```python
from build123d import *

# Parameters (mm, degrees)
F0_R     = 300
F1_DEPTH = 17.1
F3_DEPTH = 2
F4_R     = 4
F5_DEPTH = 25
F6_R     = 48
F7_DEPTH = 6
F8_R     = 15
F9_DEPTH = 11.101


# Not quite as in the source:
# - a feature names something its author has since deleted; it is built from what else it names


with BuildPart() as f1:
    # F0 (on Top) → F1 (new body)
    with BuildSketch(Plane.XY):
        Circle(F0_R)
    extrude(amount=F1_DEPTH)

    # F2 (on face) → F3 (cut)
    with BuildSketch(Plane.XY.offset(17.1)):
        Polygon((-144.8616802798, -16.1682461039), (-263.6556195192, -134.9621853432), (-134.9621853432, -263.6556195192), (-16.1682461039, -144.8616802798), align=None)
        Polygon((144.8616802798, -16.1682461039), (16.1682461039, -144.8616802798), (134.9621853432, -263.6556195192), (263.6556195192, -134.9621853432), align=None)
        Polygon((16.1682461039, 144.8616802798), (144.8616802798, 16.1682461039), (263.6556195192, 134.9621853432), (134.9621853432, 263.6556195192), align=None)
        Polygon((-144.8616802798, 16.1682461039), (-16.1682461039, 144.8616802798), (-134.9621853432, 263.6556195192), (-263.6556195192, 134.9621853432), align=None)
    extrude(amount=-F3_DEPTH, mode=Mode.SUBTRACT)

    # F4 (on face) → F5 (cut)
    with BuildSketch(Plane.XY.offset(17.1)):
        with Locations((-263.6556195192, -99.6068462839)):
            Circle(F4_R)
        with Locations((-99.6068462839, -263.6556195192)):
            Circle(F4_R)
        with Locations((99.6068462839, -263.6556195192)):
            Circle(F4_R)
        with Locations((263.6556195192, -99.6068462839)):
            Circle(F4_R)
        with Locations((263.6556195192, 99.6068462839)):
            Circle(F4_R)
        with Locations((99.6068462839, 263.6556195192)):
            Circle(F4_R)
        with Locations((-99.6068462839, 263.6556195192)):
            Circle(F4_R)
        with Locations((-263.6556195192, 99.6068462839)):
            Circle(F4_R)
    extrude(amount=-F5_DEPTH, mode=Mode.SUBTRACT)

    # F6 (on face) → F7 (cut)
    with BuildSketch(Plane.XY.offset(17.1)):
        Circle(F6_R)
    extrude(amount=-F7_DEPTH, mode=Mode.SUBTRACT)

    # F8 (on face) → F9 (cut, through all)
    with BuildSketch(Plane.XY.offset(11.1)):
        Circle(F8_R)
    extrude(amount=-F9_DEPTH, mode=Mode.SUBTRACT)


solid = f1.part
```
Geometry: final body of the model. Coordinates: model frame, mm. A direction names the side the tool comes from. Give positions to 0.01 mm unless a question says otherwise; leave off trailing zeros. Loops run counter-clockwise (first coordinate to the right, second up) from the corner with the lowest first, then second, coordinate; pieces in that order, holes last. Notation, with made-up numbers: (-18, 46.25) - (6, 46.25) arc R32 ccw to (6, 81.25) - close; hole circle Ø1 at (63, 33). An arc over 180 degrees is marked (long way). Answer as CSV lines item,"result". Start each with the question number.
(1) Pin query (flat end, axial travel): P1, Ø7, axis at x = 263.66, y = 99.61, coming from the -Z side; P2, Ø3, axis at y = -73, z = 3.5, coming from the +X side (3 decimals); P3, Ø8, axis at y = 215, z = 6, coming from the -X side; P4, Ø2, axis at x = -89, z = 15, coming from the -Y side. Return the tip coordinate at first contact, or that it passes through.
(2) Section query C-C (z = 6.5). Give the number of separate pieces and of enclosed holes in the cut face, and give its area (3 significant figures).
(3) Section query D-D (y = -200). Output: boundary loops of the cut face in (x, z).
(4) Ray query, line 1 along X through (y, z) = (-185.5, 15.25); line 2 along Y through (x, z) = (-204, 15.25); line 3 along X through (y, z) = (98, 4.5). Return the intervals inside material, ascending. Write a range as [from, to].
(5) Mould query, pull axis X, two halves, no side actions, for faces 3 (the face through (-39.054, 297.447, 8.43)), 4 (the face through (62, 4, 17.1)), 5 (the face through (205.09, -76.397, 16.114)). Classes: +X half, -X half, draft (parallel to the pull), parting line (faces both ways), or undercut.
(6) Section query A-A (y = 0). Output: boundary loops of the cut face in (x, z), and give its area (3 significant figures).
(7) Reachability of faces 1 (the face through (62, 4, 0)), 2 (the face through (74.734, -203.427, 16.114)) from +Z, -Z, +X, -X, +Y, -Y: full face, straight path, thin tool, end or side. Return the list, or none.
Worked answers:
1,P1,"passes through"
1,P2,"stops at x = 291.355"
1,P3,"stops at x = -213.26"
1,P4,"stops at y = -286.8"
2,separate pieces,"1"
2,enclosed holes,"9"
2,area,"282,000 mm^2"
3,outline,"(-223.61, 0) - (223.61, 0) - (223.61, 17.1) - (198.62, 17.1) - (198.62, 15.1) - (71.31, 15.1) - (71.31, 17.1) - (-71.31, 17.1) - (-71.31, 15.1) - (-198.62, 15.1) - (-198.62, 17.1) - (-223.61, 17.1) - close"
4,line 1,"x = [-235.77, -213.12], [-56.81, 56.81], [213.12, 235.77]"
4,line 2,"y = [-219.96, -194.62], [-75.31, 75.31], [194.62, 219.96]"
4,line 3,"x = [-283.54, -267.32], [-259.99, 259.99], [267.32, 283.54]"
5,face 3,"parting line"
5,face 4,"draft"
5,face 5,"undercut"
6,outline,"(-300, 0) - (-15, 0) - (-15, 11.1) - (-48, 11.1) - (-48, 17.1) - (-300, 17.1) - close; (15, 0) - (300, 0) - (300, 17.1) - (48, 17.1) - (48, 11.1) - (15, 11.1) - close"
6,area,"9,350 mm^2"
7,face 1,"-Z, +X, -X, +Y, -Y"
7,face 2,"+Z"
